Part model, mm, in its own coordinate system. Give positions to 0.01 mm unless a question says otherwise; leave off trailing zeros. Write each loop counter-clockwise with the first axis right and the second up, starting at its lowest first coordinate (ties: lowest second). Pieces come first, ordered by that corner, then holes. Notation, with made-up numbers: M 10,46.5 L 69,46.5 A12 cw 69,53.5 Z; hole C 4.25,-16 d9. An arc over 180 degrees is marked long. Answer as CSV lines item,"result". Start each with the question number.
Item 1: Wall check: L1, parallel to Y at x = -74.5, z = 1.5; L2, parallel to X at y = -12.5, z = -0.25; L3, parallel to X at y = -32, z = 3. Give the ranges that are in metal, low to high. Write a range as from..to.
Item 2: Band-saw the part on B-B, the plane z = -0.75. List the corners of the cut face in (x, y).
Item 3: Band-saw the part on C-C, the plane y = -37.5. List the corners of the cut face in (x, z) (3 decimals).
Item 4: Band-saw the part on A-A, the plane x = 102.5. List the corners of the cut face in (y, z) (3 decimals).
Item 5: Pin check, flat tip, straight feed: pin 1 (1.5 mm diameter, centred on x = -193, z = -1.5, fed in from -Y). Stop position of the tip, or through.
from build123d import *

# Parameters (mm, degrees)
F1_DEPTH = 3.175
F2_R     = 5.08


with BuildPart() as f1:
    # F0 (on Top) → F1 (new body, symmetric)
    with BuildSketch(Plane.XY):
        Polygon((304.414174, 0), (-305.185826, 0), (-254.385826, -50.8), (253.614174, -50.8), align=None)
    extrude(amount=F1_DEPTH, both=True)

    # F2
    f2_edges = [f1.edges().sort_by_distance(p)[0] for p in [
        (-0.385826, -50.8, -3.175),
        (-0.385826, 0, -3.175),
    ]]
    fillet(f2_edges, radius=F2_R)


solid = f1.part
Output:
1,L1,"-50.78..-0.02"
1,L2,"-292.69..291.91"
1,L3,"-273.19..272.41"
2,outline,"M -304.44,-0.75 L -255.13,-50.05 L 254.36,-50.05 L 303.67,-0.75 Z"
3,outline,"M -267.686,-3.175 L 266.914,-3.175 L 266.914,3.175 L -267.686,3.175 Z"
4,outline,"M -50.8,1.905 A5.08 ccw -45.72,-3.175 L -5.08,-3.175 A5.08 ccw 0,1.905 L 0,3.175 L -50.8,3.175 Z"
5,pin 1,"y = -50.05"
